from build123d import *

# Parameters (mm, degrees)
SKETCH1_W           = 67
SKETCH1_H           = 12
BOSS_EXTRUDE1_DEPTH = 0.75
SKETCH2_R           = 0.5
CUT_EXTRUDE1_DEPTH  = 1.5
SKETCH3_R           = 1.5
CUT_EXTRUDE2_DEPTH  = 1.5


with BuildPart() as part:
    # Sketch1 → Boss-Extrude1 (new, symmetric)
    with BuildSketch(Plane(origin=(0, 0, 0), x_dir=(0, 1, 0), z_dir=(0, 0, 1))):
        Rectangle(SKETCH1_W, SKETCH1_H)
    extrude(amount=BOSS_EXTRUDE1_DEPTH, both=True)

    # Sketch2 → Cut-Extrude1 (cut)
    with BuildSketch(Plane.XY.offset(0.75)):
        with Locations((4.5, -13)):
            Circle(SKETCH2_R)
        with Locations((4.5, -10.5)):
            Circle(SKETCH2_R)
        with Locations((4.5, -8)):
            Circle(SKETCH2_R)
        with Locations((4.5, -5.5)):
            Circle(SKETCH2_R)
        with Locations((4.5, -3)):
            Circle(SKETCH2_R)
        with Locations((4.5, -0.5)):
            Circle(SKETCH2_R)
        with Locations((4.5, 2)):
            Circle(SKETCH2_R)
        with Locations((4.5, 4.5)):
            Circle(SKETCH2_R)
        with Locations((4.5, 7)):
            Circle(SKETCH2_R)
        with Locations((4.5, 9.5)):
            Circle(SKETCH2_R)
        with Locations((4.5, 12)):
            Circle(SKETCH2_R)
    extrude(amount=-CUT_EXTRUDE1_DEPTH, mode=Mode.SUBTRACT)

    # Sketch3 → Cut-Extrude2 (cut)
    with BuildSketch(Plane.XY.offset(0.75)):
        with Locations((2.5, -19)):
            Circle(SKETCH3_R)
        with Locations((2.5, 18)):
            Circle(SKETCH3_R)
    extrude(amount=-CUT_EXTRUDE2_DEPTH, mode=Mode.SUBTRACT)


solid = part.part
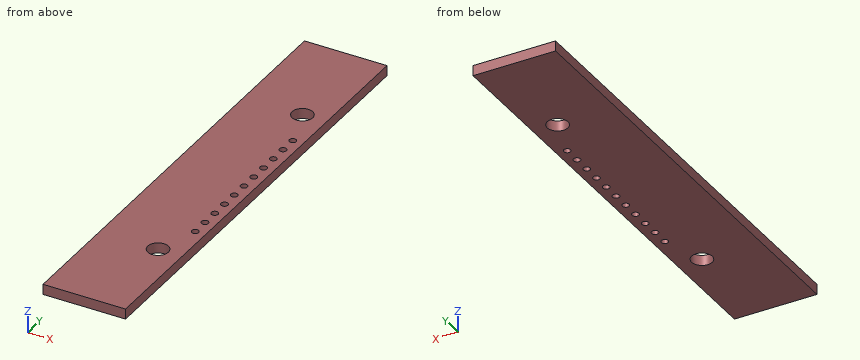
Design review of the part built by this model. Coordinates are the model's own, in mm. Coordinates: 2 decimals unless noted, no trailing zeros. Order: outer loops, then holes, each group sorted by start corner. A loop starts at its lowest first (then second) coordinate and runs counter-clockwise, first axis right, second up.
Item 1: Take a section at B-B, the plane x = 2. Write out the cut boundary in (y, z).
Item 2: Take a section at A-A, the plane z = -0.4. Count the separate pieces of the cut face and the enclosed holes in it, then the cut area to 3 significant figures.
Item 3: For line 1 (Y direction, x = 2.5, z = -0.3); line 2 (Y direction, x = 3.5, z = -0.65), list the stretches that pass through material, from the lowest coordinate up.
The answers:
1. outline: (-33.5, -0.75) - (-20.41, -0.75) - (-20.41, 0.75) - (-33.5, 0.75) - close; (-17.59, -0.75) - (16.59, -0.75) - (16.59, 0.75) - (-17.59, 0.75) - close; (19.41, -0.75) - (33.5, -0.75) - (33.5, 0.75) - (19.41, 0.75) - close
2. separate pieces: 1
2. enclosed holes: 13
2. area: 781 mm2
3. line 1: y = -33.5 to -20.5, -17.5 to 16.5, 19.5 to 33.5
3. line 2: y = -33.5 to -20.12, -17.88 to 16.88, 19.12 to 33.5
